Part model, mm, in its own coordinate system. A direction names the side the tool comes from. Coordinates: 2 decimals unless noted, no trailing zeros. Loops run counter-clockwise (first coordinate to the right, second up) from the corner with the lowest first, then second, coordinate; pieces in that order, holes last. Notation, with made-up numbers: M -7,-5.5 L 16,-5.5 A18 ccw 16,14.5 Z; hole C -22,54 d5. An arc over 180 degrees is marked long. Use a Markdown table: item, result. Add a question column.
1) Wall check: probe 1 along Z at (x, y) = (27, 3.25); probe 2 along Y at (x, z) = (25, -4.75); probe 3 along X at (y, z) = (16.5, 6). Give the ranges that are in metal, low to high. Write a range as from..to.
2) Tool access for faces 1 (the flat face through (-21.6, 7, 0.1)), 2 (the cylindrical face through (16.217, 10.866, 0.14)), 3 (the cylindrical face through (6.69, 26.08, 3.45)): list every direction of +Z, -Z, +X, -X, +Y, -Y with a clear straight run to the whole face (end or side of a thin tool).
3) Pin check, flat tips, straight feed: pin 1 Ø12 at (x, z) = (8.5, -3.5) entering from -Y; pin 2 Ø4 at (y, z) = (10.5, -4) entering from +X; pin 3 Ø11.5 at (x, z) = (27, -1) entering from +Y; pin 4 Ø5 at (y, z) = (17, -1) entering from -X. Stop position of each tip, or through.
4) Pull direction X, two halves, no side cores. Call faces 4 (the flat face through (32.5, 7, 0.1)), 5 (the flat face through (12.5, 19, 0)), 6 (the flat face through (0, 24.104, 0)): released by +X, released by -X, zero draft, split by the parting line, or undercut.
5) Band-saw the part on B-B (z = -1.5). List the corners of the cut face in (x, y), plus the area to 3 significant figures.
6) Band-saw the part on A-A (y = 5). List the corners of the cut face in (x, z), plus the area to 3 significant figures.
7) Band-saw the part on C-C (y = 9.5). List the corners of the cut face in (x, z).
8) Band-saw the part on D-D (x = 21). List the corners of the cut face in (y, z).
from build123d import *

# Parameters (mm, degrees)
F1_DEPTH = 10
F2_R     = 2.25
F3_DEPTH = 25
F4_R     = 5.25
F4_R_2   = 2.25
F5_DEPTH = 3
F6_W     = 25
F6_H     = 10
F7_DEPTH = 20
F8_R     = 1.75
F9_DEPTH = 4


with BuildPart() as f1:
    # F0 (on Top) → F1 (new body, symmetric)
    with BuildSketch(Plane.XY):
        with BuildLine():
            Line((-35, 7), (-35, 0))
            Line((-35, 0), (-14.456832, 0))
            ThreePointArc((-14.456832, 0), (0, 11), (14.456832, 0))
            Line((14.456832, 0), (35, 0))
            Line((35, 0), (35, 7))
            Line((35, 7), (19.052559, 7))
            ThreePointArc((19.052559, 7), (0, 18), (-19.052559, 7))
            Line((-19.052559, 7), (-35, 7))
        make_face()
    extrude(amount=F1_DEPTH, both=True)

    # F2 (on face) → F3 (cut)
    with BuildSketch(Plane(origin=(0, 7, 0), x_dir=(-1, 0, 0), z_dir=(0, 1, 0))):
        with Locations((-27.026279, 0)):
            Circle(F2_R)
        with Locations((27.026279, 0)):
            Circle(F2_R)
    extrude(amount=-F3_DEPTH, mode=Mode.SUBTRACT)

    # F4 (on face) → F5 (cut)
    with BuildSketch(Plane(origin=(0, 7, 0), x_dir=(-1, 0, 0), z_dir=(0, 1, 0))):
        with Locations((27.026279, 0)):
            Circle(F4_R)
        with Locations((27.026279, 0)):
            Circle(F4_R_2, mode=Mode.SUBTRACT)
        with Locations((-27.026279, 0)):
            Circle(F4_R)
    extrude(amount=-F5_DEPTH, mode=Mode.SUBTRACT)

    # F6 (on face) → F7 (join)
    with BuildSketch(Plane.XY.offset(10)):
        with Locations((0, 19.103867)):
            Rectangle(F6_W, F6_H)
    extrude(amount=-F7_DEPTH)

    # F8 (on face) → F9 (join)
    with BuildSketch(Plane(origin=(0, 24.103867, 0), x_dir=(-1, 0, 0), z_dir=(0, 1, 0))):
        with Locations((7.5, -5)):
            Circle(F8_R)
        with Locations((-7.5, -5)):
            Circle(F8_R)
        with Locations((7.5, 5)):
            Circle(F8_R)
        with Locations((-7.5, 5)):
            Circle(F8_R)
    extrude(amount=F9_DEPTH)


solid = f1.part
Entries:
| question | item | result |
|---|---|---|
| 1 | probe 1 | -10..-2.25, 2.25..10 |
| 1 | probe 2 | 0..4 |
| 1 | probe 3 | -12.5..12.5 |
| 2 | face 1 | +Z, -Z, -X, +Y |
| 2 | face 2 | +Z, -Z, +X, +Y |
| 2 | face 3 | +Y |
| 3 | pin 1 | y = 0 |
| 3 | pin 2 | x = 18.1 |
| 3 | pin 3 | y = 7 |
| 3 | pin 4 | x = -12.5 |
| 4 | face 4 | zero draft |
| 4 | face 5 | released by +X |
| 4 | face 6 | undercut |
| 5 | outline | M -35,0 L -28.7,0 L -28.7,4 L -32.06,4 L -32.06,7 L -35,7 Z; M -25.35,0 L -14.46,0 A15 cw 14.46,0 L 25.35,0 L 25.35,4 L 22,4 L 22,7 L 19.05,7 A22 ccw 12.5,14.1 L 12.5,24.1 L -12.5,24.1 L -12.5,14.1 A22 ccw -19.05,7 L -22,7 L -22,4 L -25.35,4 Z; M 28.7,0 L 35,0 L 35,7 L 32.06,7 L 32.06,4 L 28.7,4 Z |
| 5 | area | 649 mm2 |
| 6 | outline | M -35,-10 L -12,-10 L -12,10 L -35,10 Z; M 12,-10 L 35,-10 L 35,10 L 12,10 Z; hole C -27.03,0 d10.5; hole C 27.03,0 d10.5 |
| 6 | area | 747 mm2 |
| 7 | outline | M -17.37,-10 L -6.54,-10 L -6.54,10 L -17.37,10 Z; M 6.54,-10 L 17.37,-10 L 17.37,10 L 6.54,10 Z |
| 8 | outline | M 0,-10 L 7,-10 L 7,10 L 0,10 Z |
